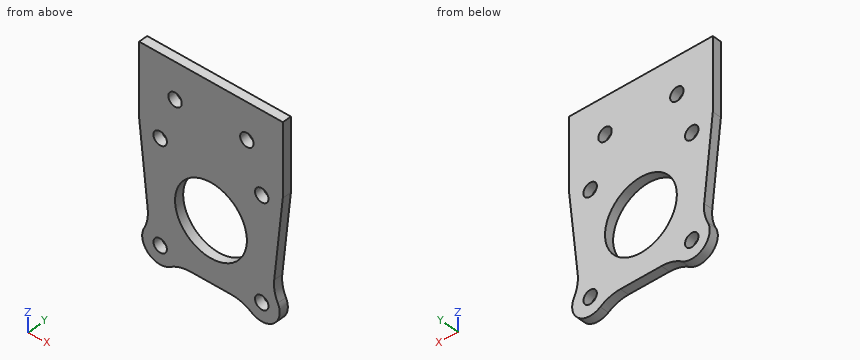
```python
from build123d import *

# Parameters (mm, degrees)
BOSS_EXTRUDE1_DEPTH            = 3.175
F_1_1_DIAMETER_HOLE1_D         = 25.4
SKETCH6_R                      = 2.38125
CUT_EXTRUDE1_DEPTH             = 63.666104275
SKETCH7_R                      = 6.35
SKETCH7_R_2                    = 2.38125
BOSS_EXTRUDE2_DEPTH            = 3.175
F_3_16_0_1875_DIAMETER_HOLE1_D = 4.7625
FILLET1_R                      = 12.7


with BuildPart() as part:
    # Sketch1 → Boss-Extrude1 (new body)
    with BuildSketch(Plane(origin=(0, 0, 0), x_dir=(1, 0, 0), z_dir=(0, 1, 0))):
        Polygon((0, 42), (-42, 42), (-46.4, 0), (-46.4, -25.4), (4.4, -25.4), (4.4, 0), align=None)
    extrude(amount=BOSS_EXTRUDE1_DEPTH)

    # 1 (1) Diameter Hole1 (through all)
    with Locations(Plane(origin=(0, 3.175, 0), x_dir=(1, 0, 0), z_dir=(0, 1, 0))):
        with Locations((-21, 21)):
            Hole(F_1_1_DIAMETER_HOLE1_D / 2)

    # Sketch6 → Cut-Extrude1 (cut, through all)
    with BuildSketch(Plane(origin=(0, 3.175, 0), x_dir=(1, 0, 0), z_dir=(0, 1, 0))):
        with Locations(Location((-38.960512242, 38.960512242, 0), (0, 0, 270))):
            Circle(SKETCH6_R)
        with Locations(Location((-38.960512242, 3.039487758, 0), (0, 0, 270))):
            Circle(SKETCH6_R)
        with Locations(Location((-3.039487758, 3.039487758, 0), (0, 0, 270))):
            Circle(SKETCH6_R)
        with Locations(Location((-3.039487758, 38.960512242, 0), (0, 0, 270))):
            Circle(SKETCH6_R)
    extrude(amount=-CUT_EXTRUDE1_DEPTH, mode=Mode.SUBTRACT)

    # Sketch7 → Boss-Extrude2 (add)
    # profile 1 of 2: a face of its own
    with BuildSketch(Plane(origin=(0, 3.175, 0), x_dir=(1, 0, 0), z_dir=(0, 1, 0))):
        with Locations((-38.960512242, 38.960512242)):
            Circle(SKETCH7_R)
        with Locations(Location((-38.960512242, 38.960512242, 0), (0, 0, 270))):
            Circle(SKETCH7_R_2, mode=Mode.SUBTRACT)
    # profile 2 of 2: a face of its own
    with BuildSketch(Plane(origin=(0, 3.175, 0), x_dir=(1, 0, 0), z_dir=(0, 1, 0))):
        with Locations((-3.039487758, 38.960512242)):
            Circle(SKETCH7_R)
        with Locations(Location((-3.039487758, 38.960512242, 0), (0, 0, 270))):
            Circle(SKETCH7_R_2, mode=Mode.SUBTRACT)
    extrude(amount=-BOSS_EXTRUDE2_DEPTH)

    # 3/16 (0.1875) Diameter Hole1 (through all)
    with Locations(Plane(origin=(0, 3.175, 0), x_dir=(1, 0, 0), z_dir=(0, 1, 0))):
        with Locations((-33.7, -12.7), (-8.3, -12.7)):
            Hole(F_3_16_0_1875_DIAMETER_HOLE1_D / 2)

    # Fillet1
    fillet1_edges = [part.edges().sort_by_distance(p)[0] for p in [
        (-42.844694729, 1.5875, -33.937004861),
        (-33.385208289, 1.5875, -42),
        (0.844694729, 1.5875, -33.937004861),
        (-8.614791711, 1.5875, -42),
    ]]
    fillet(fillet1_edges, radius=FILLET1_R)


solid = part.part
```
Geometry check sheet. Reference: the model listing, model coordinates, mm. Coordinates: 2 decimals unless noted, no trailing zeros. Order: outer loops, then holes, each group sorted by start corner. A loop starts at its lowest first (then second) coordinate and runs counter-clockwise, first axis right, second up. Notation, with made-up numbers: (-38, 65.25) - (-15, 65.25) arc R26 cw to (-15, 97.25) - close; hole circle Ø1 at (1, 1). An arc over 180 degrees is marked (long way). Answer in a Markdown table with one row per item. Add a question column.
1. Material ranges on L1, parallel to X at y = 1.6, z = 12.7; L2, parallel to X at y = 0.8, z = -40.5; L3, parallel to Z at x = -37, y = 1.5, recorded low to high. Write a range as [from, to].
2. Section check A-A (x = -21). Enter the section's corners in (y, z) (3 decimals), plus the area to 3 significant figures.
3. Gauge pin test, flat end, axial feed: pin 1 Ø5.5 at (x, z) = (-38.96, -3.04) entering from -Y. Record the tip position at first contact, or that the pin passes through.
4. Section check D-D (y = 2.6). Enter the section's corners in (x, z), plus the area to 3 significant figures.
5. Section check C-C (z = 12.7). Enter the section's corners in (x, y) (3 decimals).
6. Section check B-B (z = -21). Enter the section's corners in (x, y) (3 decimals), plus the area to 3 significant figures.
Data:
| question | item | result |
|---|---|---|
| 1 | L1 | x = [-46.4, -36.08], [-31.32, -10.68], [-5.92, 4.4] |
| 1 | L2 | x = [-45.12, -40.78], [-37.14, -4.86], [-1.22, 3.12] |
| 1 | L3 | z = [-45, -40.31], [-37.61, -4.39], [-1.69, 25.4] |
| 2 | outline | (0, -42) - (3.175, -42) - (3.175, -33.7) - (0, -33.7) - close; (0, -8.3) - (3.175, -8.3) - (3.175, 25.4) - (0, 25.4) - close |
| 2 | area | 133 mm² |
| 3 | pin 1 | stops at y = 0 |
| 4 | outline | (-46.4, 0) - (-43.35, -29.09) arc R12.7 cw to (-44.63, -36.11) arc R6.35 ccw to (-35.38, -44.21) arc R12.7 cw to (-28.23, -42) - (-13.77, -42) arc R12.7 cw to (-6.62, -44.21) arc R6.35 ccw to (2.63, -36.11) arc R12.7 cw to (1.35, -29.09) - (4.4, 0) - (4.4, 25.4) - (-46.4, 25.4) - close; hole circle Ø4.76 at (-38.96, -38.96); hole circle Ø4.76 at (-38.96, -3.04); hole circle Ø4.76 at (-33.7, 12.7); hole circle Ø25.4 at (-21, -21); hole circle Ø4.76 at (-8.3, 12.7); hole circle Ø4.76 at (-3.04, -38.96); hole circle Ø4.76 at (-3.04, -3.04) |
| 4 | area | 2,720 mm² |
| 5 | outline | (-46.4, 0) - (-36.081, 0) - (-36.081, 3.175) - (-46.4, 3.175) - close; (-31.319, 0) - (-10.681, 0) - (-10.681, 3.175) - (-31.319, 3.175) - close; (-5.919, 0) - (4.4, 0) - (4.4, 3.175) - (-5.919, 3.175) - close |
| 6 | outline | (-44.2, 0) - (-33.7, 0) - (-33.7, 3.175) - (-44.2, 3.175) - close; (-8.3, 0) - (2.2, 0) - (2.2, 3.175) - (-8.3, 3.175) - close |
| 6 | area | 66.7 mm² |
